Verification items for the finished model (mm, model axes). Face numbers are marked on the shaded views. Give positions to 0.01 mm unless a question says otherwise; leave off trailing zeros. Loops run counter-clockwise (first coordinate to the right, second up) from the corner with the lowest first, then second, coordinate; pieces in that order, holes last. Notation, with made-up numbers: M 46.25,13.25 L 73.25,13.25 A23 ccw 73.25,44.25 Z; hole C -19.75,-15 d10. An arc over 180 degrees is marked long. Write each question's results on one line, items separated by ' | '. Start each with the question number.
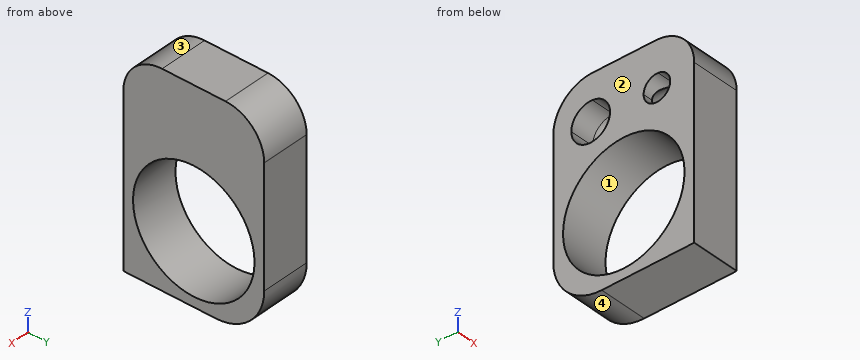
```python
from build123d import *

# Parameters (mm, degrees)
F0_R     = 12.55
F1_DEPTH = 5
F2_DEPTH = 5
F3_R     = 10


with BuildPart() as f1:
    # F0 (on Right) → F1 (new body)
    with BuildSketch(Plane.YZ):
        with BuildLine():
            ThreePointArc((14.55, 20), (12.2068542495, 25.6568542495), (6.55, 28))
            Line((6.55, 28), (-6.55, 28))
            ThreePointArc((-6.55, 28), (-12.2068542495, 25.6568542495), (-14.55, 20))
            Line((-14.55, 20), (-14.55, -14.55))
            Line((-14.55, -14.55), (14.55, -14.55))
            Line((14.55, -14.55), (14.55, 20))
        make_face()
        Circle(F0_R, mode=Mode.SUBTRACT)
        with BuildLine():
            Line((2.8404028665, 18.7938524157), (-4.0904028665, 18.7938524157))
            ThreePointArc((-4.0904028665, 18.7938524157), (-6.8404028665, 16.0438524157), (-9.5904028665, 18.7938524157))
            ThreePointArc((-9.5904028665, 18.7938524157), (-8.8718404378, 20.6474331111), (-7.0916673072, 21.5323494818))
            Line((-7.0916673072, 21.5323494818), (6.4749272755, 22.7771208717))
            ThreePointArc((6.4749272755, 22.7771208717), (9.5365202263, 21.748670715), (10.8404028665, 18.7938524157))
            ThreePointArc((10.8404028665, 18.7938524157), (6.8404028665, 14.7938524157), (2.8404028665, 18.7938524157))
        make_face(mode=Mode.SUBTRACT)
        with BuildLine():
            ThreePointArc((-7.0916673072, 21.5323494818), (-4.9868221712, 20.825289987), (-4.0904028665, 18.7938524157))
            Line((-4.0904028665, 18.7938524157), (2.8404028665, 18.7938524157))
            ThreePointArc((2.8404028665, 18.7938524157), (3.8855845672, 21.4899697755), (6.4749272755, 22.7771208717))
            Line((6.4749272755, 22.7771208717), (-7.0916673072, 21.5323494818))
        make_face()
    extrude(amount=-F1_DEPTH)

    # F0 (on Right) → F2 (join)
    with BuildSketch(Plane.YZ):
        with BuildLine():
            ThreePointArc((14.55, 20), (12.2068542495, 25.6568542495), (6.55, 28))
            Line((6.55, 28), (-6.55, 28))
            ThreePointArc((-6.55, 28), (-12.2068542495, 25.6568542495), (-14.55, 20))
            Line((-14.55, 20), (-14.55, -14.55))
            Line((-14.55, -14.55), (14.55, -14.55))
            Line((14.55, -14.55), (14.55, 20))
        make_face()
        Circle(F0_R, mode=Mode.SUBTRACT)
        with BuildLine():
            Line((2.8404028665, 18.7938524157), (-4.0904028665, 18.7938524157))
            ThreePointArc((-4.0904028665, 18.7938524157), (-6.8404028665, 16.0438524157), (-9.5904028665, 18.7938524157))
            ThreePointArc((-9.5904028665, 18.7938524157), (-8.8718404378, 20.6474331111), (-7.0916673072, 21.5323494818))
            Line((-7.0916673072, 21.5323494818), (6.4749272755, 22.7771208717))
            ThreePointArc((6.4749272755, 22.7771208717), (9.5365202263, 21.748670715), (10.8404028665, 18.7938524157))
            ThreePointArc((10.8404028665, 18.7938524157), (6.8404028665, 14.7938524157), (2.8404028665, 18.7938524157))
        make_face(mode=Mode.SUBTRACT)
        with BuildLine():
            ThreePointArc((-9.5904028665, 18.7938524157), (-6.8404028665, 16.0438524157), (-4.0904028665, 18.7938524157))
            Line((-4.0904028665, 18.7938524157), (-9.5904028665, 18.7938524157))
        make_face()
        with BuildLine():
            Line((-9.5904028665, 18.7938524157), (-4.0904028665, 18.7938524157))
            ThreePointArc((-4.0904028665, 18.7938524157), (-4.9868221712, 20.825289987), (-7.0916673072, 21.5323494818))
            ThreePointArc((-7.0916673072, 21.5323494818), (-8.8718404378, 20.6474331111), (-9.5904028665, 18.7938524157))
        make_face()
        with BuildLine():
            ThreePointArc((-7.0916673072, 21.5323494818), (-4.9868221712, 20.825289987), (-4.0904028665, 18.7938524157))
            Line((-4.0904028665, 18.7938524157), (2.8404028665, 18.7938524157))
            ThreePointArc((2.8404028665, 18.7938524157), (3.8855845672, 21.4899697755), (6.4749272755, 22.7771208717))
            Line((6.4749272755, 22.7771208717), (-7.0916673072, 21.5323494818))
        make_face()
        with BuildLine():
            ThreePointArc((6.4749272755, 22.7771208717), (3.8855845672, 21.4899697755), (2.8404028665, 18.7938524157))
            Line((2.8404028665, 18.7938524157), (10.8404028665, 18.7938524157))
            ThreePointArc((10.8404028665, 18.7938524157), (9.5365202263, 21.748670715), (6.4749272755, 22.7771208717))
        make_face()
        with BuildLine():
            Line((10.8404028665, 18.7938524157), (2.8404028665, 18.7938524157))
            ThreePointArc((2.8404028665, 18.7938524157), (6.8404028665, 14.7938524157), (10.8404028665, 18.7938524157))
        make_face()
    extrude(amount=F2_DEPTH)

    # F3
    f3_edges = [f1.edges().sort_by_distance(p)[0] for p in [
        (0, 14.55, -14.55),
    ]]
    fillet(f3_edges, radius=F3_R)

    # F0 (on Right) → F4 (revolve, cut)
    with BuildSketch(Plane.YZ):
        with BuildLine():
            Line((-9.5904028665, 18.7938524157), (-4.0904028665, 18.7938524157))
            ThreePointArc((-4.0904028665, 18.7938524157), (-4.9868221712, 20.825289987), (-7.0916673072, 21.5323494818))
            ThreePointArc((-7.0916673072, 21.5323494818), (-8.8718404378, 20.6474331111), (-9.5904028665, 18.7938524157))
        make_face()
        with BuildLine():
            ThreePointArc((-7.0916673072, 21.5323494818), (-4.9868221712, 20.825289987), (-4.0904028665, 18.7938524157))
            Line((-4.0904028665, 18.7938524157), (2.8404028665, 18.7938524157))
            ThreePointArc((2.8404028665, 18.7938524157), (3.8855845672, 21.4899697755), (6.4749272755, 22.7771208717))
            Line((6.4749272755, 22.7771208717), (-7.0916673072, 21.5323494818))
        make_face()
        with BuildLine():
            ThreePointArc((6.4749272755, 22.7771208717), (3.8855845672, 21.4899697755), (2.8404028665, 18.7938524157))
            Line((2.8404028665, 18.7938524157), (10.8404028665, 18.7938524157))
            ThreePointArc((10.8404028665, 18.7938524157), (9.5365202263, 21.748670715), (6.4749272755, 22.7771208717))
        make_face()
    revolve(axis=Axis((0, 0.625, 18.7938524157), (0, 1, 0)), mode=Mode.SUBTRACT)


solid = f1.part
```
1. Release check for a two-part mould opening along Y. For the marked faces 1, 2, 3 and 4 record: released by +Y, released by -Y, zero draft, split by the parting line, or undercut.
2. Thickness scan on probe 1 along Z at (x, y) = (-0.75, -8); probe 2 along Z at (x, y) = (-3, -7.25); probe 3 along Y at (x, z) = (-1, 0.5). Record the ranges inside material, lowest first.
3. Section check A-A, the plane z = 0. Record the boundary of the cut face in (x, y), plus the area to 3 significant figures.
4. Depth check by flat-ended pin: pin 1 Ø1 at (x, z) = (-1, -7) entering from +Y. Enter the tip coordinate at first touch or a pass-through.
5. Section check B-B, the plane y = 0. Record the boundary of the cut face in (x, z), plus the area to 3 significant figures.
6. Section check C-C, the plane y = -9. Record the boundary of the cut face in (x, z).
7. Section check D-D, the plane z = 8. Record the boundary of the cut face in (x, y), plus the area to 3 significant figures.
Filled sheet:
1) face 1: undercut | face 2: zero draft | face 3: released by -Y | face 4: released by +Y
2) probe 1: -14.55 to -9.67, 9.67 to 16.3, 21.29 to 27.87 | probe 2: -14.55 to -10.24, 10.24 to 16.07, 21.51 to 27.97 | probe 3: -14.55 to -12.54, 12.54 to 14.55
3) outline: M -5,-14.55 L 5,-14.55 L 5,-12.55 L -5,-12.55 Z; M -5,12.55 L 5,12.55 L 5,14.55 L -5,14.55 Z | area: 40.0 mm2
4) pin 1: y = 14.36
5) outline: M -5,-14.55 L 5,-14.55 L 5,-12.55 L -5,-12.55 Z; M -5,12.55 L 5,12.55 L 5,28 L -5,28 Z; hole C 0,18.79 d6.78 | area: 138 mm2
6) outline: M -5,-14.55 L 5,-14.55 L 5,-8.75 L -5,-8.75 Z; M -5,8.75 L 5,8.75 L 5,27.62 L -5,27.62 L -5,20.5 L 0,20.5 A1.7 cw 0,17.09 L -5,17.09 Z
7) outline: M -5,-14.55 L 5,-14.55 L 5,-9.67 L -5,-9.67 Z; M -5,9.67 L 5,9.67 L 5,14.55 L -5,14.55 Z | area: 97.6 mm2
